Part model, mm, in its own coordinate system. Face numbers are marked on the shaded views. A direction names the side the tool comes from. Give positions to 0.01 mm unless a question says otherwise; leave off trailing zeros. Write each loop counter-clockwise with the first axis right and the second up, starting at its lowest first coordinate (ties: lowest second). Pieces come first, ordered by that corner, then holes. Notation, with made-up numbers: (62, 3) - (80, 3) arc R28 ccw to (80, 38) - close; hole circle Ø5 at (34.25, -11.75). An arc over 180 degrees is marked (long way). Answer in a Markdown table with one row per item. Add a question column.
1. Which spindle directions (+Z, -Z, +X, -X, +Y, -Y) get a long thin tool onto all of the face, cutting with end or side? Do the marked faces 4, 5 and 6. Say none if no direction does.
2. Probe line 1 along Y through (x, z) = (0, 35.2); line 2 along Y through (x, z) = (0, 34.75); line 3 along X through (y, z) = (-1.5, 26). List the from-to ranges inside material, lowest first.
3. Drop flat-ended pins along their axis: pin 1 Ø1.8 at (x, y) = (-0.5, -0.5) entering from +Z; pin 2 Ø1.5 at (x, y) = (0.5, 0.5) entering from +Z; pin 3 Ø2 at (y, z) = (0, 8.5) entering from +X. Give the stop position or say it passes through.
4. Band-saw the part on A-A on z = 13.5. Write the cut outline in (x, y).
5. Pull direction X, two halves, no side cores. Call the marked faces 1, 2 and 3: released by +X, released by -X, zero draft, split by the parting line, or undercut.
```python
from build123d import *

# Parameters (mm, degrees)
ESBO_O1_W                = 69
ESBO_O1_H                = 8.5
RESSALTO_EXTRUS_O1_DEPTH = 6
ESBO_O2_W                = 50
ESBO_O2_H                = 8.5
RESSALTO_EXTRUS_O2_DEPTH = 30
ESBO_O3_R                = 2.5
CORTE_EXTRUS_O1_DEPTH    = 7
FILETE1_R                = 4
ESBO_O4_R                = 3
CORTE_EXTRUS_O2_DEPTH    = 1
ESBO_O5_R                = 1.5
CORTE_EXTRUS_O3_DEPTH    = 1
ESBO_O6_R                = 0.5
CORTE_EXTRUS_O4_DEPTH    = 1


with BuildPart() as part:
    # Esboço1 → Ressalto-extrusão1 (new body)
    with BuildSketch(Plane.XY):
        Rectangle(ESBO_O1_W, ESBO_O1_H)
    extrude(amount=RESSALTO_EXTRUS_O1_DEPTH)

    # Esboço2 → Ressalto-extrusão2 (add)
    with BuildSketch(Plane.XY.offset(6)):
        Rectangle(ESBO_O2_W, ESBO_O2_H)
    extrude(amount=RESSALTO_EXTRUS_O2_DEPTH)

    # Esboço3 → Corte-extrusão1 (cut, through all)
    with BuildSketch(Plane.XY.offset(6)):
        with Locations((-30.25, 0)):
            Circle(ESBO_O3_R)
        with Locations((30.25, 0)):
            Circle(ESBO_O3_R)
    extrude(amount=-CORTE_EXTRUS_O1_DEPTH, mode=Mode.SUBTRACT)

    # Filete1
    filete1_edges = [part.edges().sort_by_distance(p)[0] for p in [
        (-34.5, 4.25, 3),
        (34.5, 4.25, 3),
        (34.5, -4.25, 3),
        (-34.5, -4.25, 3),
    ]]
    fillet(filete1_edges, radius=FILETE1_R)

    # Esboço4 → Corte-extrusão2 (cut)
    with BuildSketch(Plane.XY.offset(36)):
        Circle(ESBO_O4_R)
    extrude(amount=-CORTE_EXTRUS_O2_DEPTH, mode=Mode.SUBTRACT)

    # Esboço5 → Corte-extrusão3 (cut)
    with BuildSketch(Plane.XY.offset(35)):
        Circle(ESBO_O5_R)
    extrude(amount=-CORTE_EXTRUS_O3_DEPTH, mode=Mode.SUBTRACT)

    # Esboço6 → Corte-extrusão4 (cut)
    with BuildSketch(Plane.XY.offset(34)):
        Circle(ESBO_O6_R)
    extrude(amount=-CORTE_EXTRUS_O4_DEPTH, mode=Mode.SUBTRACT)


solid = part.part
```
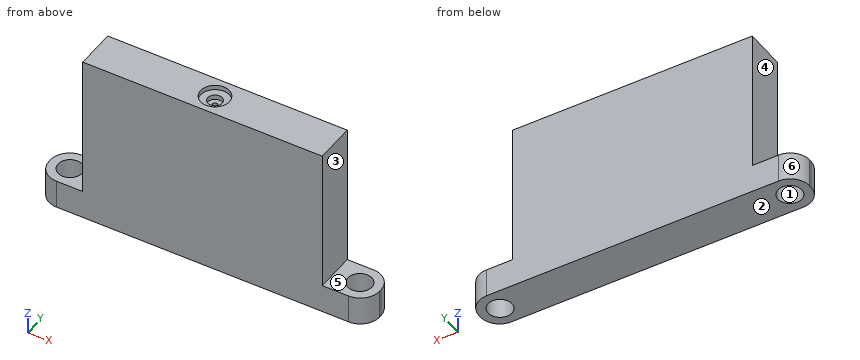
Values:
| question | item | result |
|---|---|---|
| 1 | face 4 | +Z, -X, +Y, -Y |
| 1 | face 5 | +Z, +X, +Y, -Y |
| 1 | face 6 | +Z, -Z, -X, +Y |
| 2 | line 1 | y = -4.25 to -3, 3 to 4.25 |
| 2 | line 2 | y = -4.25 to -1.5, 1.5 to 4.25 |
| 2 | line 3 | x = -25 to 25 |
| 3 | pin 1 | stops at z = 35 |
| 3 | pin 2 | stops at z = 34 |
| 3 | pin 3 | stops at x = 25 |
| 4 | outline | (-25, -4.25) - (25, -4.25) - (25, 4.25) - (-25, 4.25) - close |
| 5 | face 1 | undercut |
| 5 | face 2 | zero draft |
| 5 | face 3 | released by +X |
